Design review of the part built by this model. Coordinates are the model's own, in mm. Face numbers are marked on the shaded views. A direction names the side the tool comes from. Round coordinates to 2 decimals unless told otherwise and drop trailing zeros. Order: outer loops, then holes, each group sorted by start corner. A loop starts at its lowest first (then second) coordinate and runs counter-clockwise, first axis right, second up. Notation, with made-up numbers: (37, 35.25) - (62, 35.25) arc R20 ccw to (62, 58.25) - close; hole circle Ø5 at (25, -21). An arc over 180 degrees is marked (long way). Write item = value, one per line.
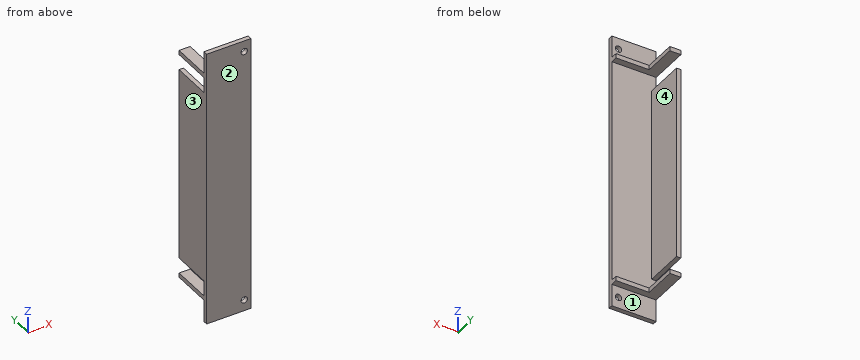
from build123d import *

# Parameters (mm, degrees)
BOSS_EXTRUDE1_DEPTH    = 126
SKETCH2_W              = 7
SKETCH2_H              = 18
SKETCH2_W_2            = 10
CUT_EXTRUDE1_DEPTH     = 130.135587659
BOSS_EXTRUDE2_DEPTH    = 2
M2_5_CLEARANCE_HOLE1_D = 2.9


with BuildPart() as part:
    # Sketch1 → Boss-Extrude1 (new body)
    with BuildSketch(Plane.XY):
        Polygon((-10, 0), (10, 0), (10, 2), (-8, 2), (-8, 20), (-10, 20), align=None)
    extrude(amount=BOSS_EXTRUDE1_DEPTH)

    # Sketch2 → Cut-Extrude1 (cut, through all)
    with BuildSketch(Plane.ZY.offset(10)):
        with Locations((15.5, 11)):
            Rectangle(SKETCH2_W, SKETCH2_H)
        with Locations((110.5, 11)):
            Rectangle(SKETCH2_W, SKETCH2_H)
        with Locations((5, 11)):
            Rectangle(SKETCH2_W_2, SKETCH2_H)
        with Locations((121, 11)):
            Rectangle(SKETCH2_W_2, SKETCH2_H)
    extrude(amount=-CUT_EXTRUDE1_DEPTH, mode=Mode.SUBTRACT)

    # Sketch3 → Boss-Extrude2 (add)
    with BuildSketch(Plane.XY.offset(116)):
        Polygon((-10, 20), (-5, 20), (-5, 5), (10, 5), (10, 2), (-5, 2), (-10, 2), align=None)
    boss_extrude2 = extrude(amount=-BOSS_EXTRUDE2_DEPTH)

    # M2.5 Clearance Hole1 (through all)
    with Locations(Plane(origin=(0, 2, 0), x_dir=(1, 0, 0), z_dir=(0, 1, 0))):
        with Locations((7, -121)):
            m2_5_clearance_hole1 = Hole(M2_5_CLEARANCE_HOLE1_D / 2)

    # Mirror1: Boss-Extrude2, M2.5 Clearance Hole1 across plane
    add(boss_extrude2.mirror(Plane.XY.offset(63)))
    add(m2_5_clearance_hole1.mirror(Plane.XY.offset(63)), mode=Mode.SUBTRACT)


solid = part.part
1) The part is to be moulded in two halves that separate along Z. For the marked faces 3 and 4, say which applies: released by +Z, released by -Z, zero draft, split by the parting line, or undercut.
Findings:
face_3 = zero draft
face_4 = undercut
2) To check wall thickness, follow L1, parallel to Z at x = 7, y = 0.8; L2, parallel to X at y = 0.9, z = 5; L3, parallel to Z at x = -7.5, y = 3.25. State the ranges of each line that lie inside material, in increasing order. Write a range as from..to.
Findings:
L1 = 0..3.55, 6.45..119.55, 122.45..126
L2 = -10..5.55, 8.45..10
L3 = 10..12, 114..116
3) We need section B-B on z = 5. Write out the cut boundary in (x, y), and give its area (3 significant figures).
Findings:
outline = (-10, 0) - (5.55, 0) - (5.55, 2) - (-10, 2) - close; (8.45, 0) - (10, 0) - (10, 2) - (8.45, 2) - close
area = 34.2 mm^2
4) We need section A-A on x = 7. Write out the cut boundary in (y, z).
Findings:
outline = (0, 0) - (2, 0) - (2, 3.55) - (0, 3.55) - close; (0, 6.45) - (2, 6.45) - (2, 10) - (5, 10) - (5, 12) - (2, 12) - (2, 114) - (5, 114) - (5, 116) - (2, 116) - (2, 119.55) - (0, 119.55) - close; (0, 122.45) - (2, 122.45) - (2, 126) - (0, 126) - close
5) For the marked faces 1 and 2, list the 3-axis set-ups (+Z, -Z, +X, -X, +Y, -Y) from which the entire face can be reached by the end or side of a thin tool; tool diameter is ignored.
Findings:
face_1 = -Z, +X, -X, +Y
face_2 = +Z, -Z, +X, -X, -Y
6) Clearance check with flat-ended pins moving along their axes: pin 1 Ø1 at (y, z) = (16.5, 98) entering from +X; pin 2 Ø10 at (x, z) = (-3.5, 81) entering from -Y; pin 3 Ø0.6 at (y, z) = (9, 115) entering from +X; pin 4 Ø1 at (x, y) = (-9, 14) entering from -Z. State where each tip first meets the part, or that it passes through.
Findings:
pin_1 = -8
pin_2 = 0
pin_3 = -5
pin_4 = 10
7) We need section C-C on z = 34. Write out the cut boundary in (x, y), and give its area (3 significant figures).
Findings:
outline = (-10, 0) - (10, 0) - (10, 2) - (-8, 2) - (-8, 20) - (-10, 20) - close
area = 76.0 mm^2
8) We need section D-D on x = 0.75. Write out the cut boundary in (y, z), and give its area (3 significant figures).
Findings:
outline = (0, 0) - (2, 0) - (2, 10) - (5, 10) - (5, 12) - (2, 12) - (2, 114) - (5, 114) - (5, 116) - (2, 116) - (2, 126) - (0, 126) - close
area = 264 mm^2
